Source: CAD feature listing. Evaluate the final solid. Frame: model axes, mm. Round coordinates to 2 decimals unless told otherwise and drop trailing zeros. Write each loop counter-clockwise with the first axis right and the second up, starting at its lowest first coordinate (ties: lowest second). Pieces come first, ordered by that corner, then holes. Notation, with made-up numbers: M -19.5,55.25 L 10.5,55.25 A34 cw 10.5,94.25 Z; hole C 36,47 d2. An arc over 180 degrees is marked long. Answer in a Markdown table with one row per item. Add a question column.
Item 1: Material intervals for probe 1 along X at (y, z) = (1.75, 249); probe 2 along X at (y, z) = (2.4, 26); probe 3 along X at (y, z) = (0.55, -40), sorted ascending.
Item 2: Cut plane D-D on x = 187.5. Return loops of the section in (y, z), and give its area (3 significant figures).
Item 3: Contact query for a flat-ended pin moving along its axis: pin 1 (1.5 mm diameter, centred on x = 364.5, y = 0.5, fed in from -Z). Output: stop coordinate, or through.
Item 4: Cut plane B-B on x = 463. Return loops of the section in (y, z).
Item 5: Mould query, pull axis X, two halves, no side actions, for faces 1 (the face through (19.52, 2.03, 62)), 2 (the face through (271.15, 1.972, 478.537)), 3 (the face through (-271.15, 1.972, -478.537)). Classes: released by +X, released by -X, zero draft, split by the parting line, or undercut.
Item 6: Cut plane A-A on z = 0. Return loops of the section in (x, y).
Item 7: Cut plane C-C on y = 0.95. Give the number of separate pieces and of enclosed holes in the cut face, and give its area (3 significant figures).
from build123d import *

# Parameters (mm, degrees)
BOSS_EXTRUDE1_DEPTH = 4
CUT_EXTRUDE1_REACH  = 842.148
SKETCH3_R           = 4
CUT_EXTRUDE2_REACH  = 842.148
SKETCH4_R           = 3.1
CIRPATTERN1_COUNT   = 6
CUT_EXTRUDE3_REACH  = 842.148
SKETCH5_R           = 65


with BuildPart() as part:
    # Sketch1 → Boss-Extrude1 (new body)
    with BuildSketch(Plane(origin=(0, 0, 0), x_dir=(1, 0, 0), z_dir=(0, 1, 0))):
        Polygon((0, 635.085296109), (-550, 317.542648054), (-550, -317.542648054), (0, -635.085296109), (550, -317.542648054), (550, 317.542648054), align=None)
    extrude(amount=BOSS_EXTRUDE1_DEPTH)

    # Sketch3 → Cut-Extrude1 (cut, up to next)
    with BuildSketch(Plane(origin=(0, 4, 0), x_dir=(1, 0, 0), z_dir=(0, 1, 0)), mode=Mode.PRIVATE) as cut_extrude1_sk1:
        with Locations(Location((53.101090522, 102.006245815, 0), (0, 0, 270))):
            Circle(SKETCH3_R)
    cut_extrude1_tool1 = extrude(cut_extrude1_sk1.sketch, amount=-CUT_EXTRUDE1_REACH, mode=Mode.PRIVATE) & part.part
    # Sketch3 → Cut-Extrude1 (cut, up to next)
    with BuildSketch(Plane(origin=(0, 4, 0), x_dir=(1, 0, 0), z_dir=(0, 1, 0)), mode=Mode.PRIVATE) as cut_extrude1_sk2:
        with Locations(Location((109.677449336, 34.581166943, 0), (0, 0, 270))):
            Circle(SKETCH3_R)
    cut_extrude1_tool2 = extrude(cut_extrude1_sk2.sketch, amount=-CUT_EXTRUDE1_REACH, mode=Mode.PRIVATE) & part.part
    # Sketch3 → Cut-Extrude1 (cut, up to next)
    with BuildSketch(Plane(origin=(0, 4, 0), x_dir=(1, 0, 0), z_dir=(0, 1, 0)), mode=Mode.PRIVATE) as cut_extrude1_sk3:
        with Locations(Location((102.006245815, -53.101090522, 0), (0, 0, 270))):
            Circle(SKETCH3_R)
    cut_extrude1_tool3 = extrude(cut_extrude1_sk3.sketch, amount=-CUT_EXTRUDE1_REACH, mode=Mode.PRIVATE) & part.part
    # Sketch3 → Cut-Extrude1 (cut, up to next)
    with BuildSketch(Plane(origin=(0, 4, 0), x_dir=(1, 0, 0), z_dir=(0, 1, 0)), mode=Mode.PRIVATE) as cut_extrude1_sk4:
        with Locations(Location((34.581166943, -109.677449336, 0), (0, 0, 270))):
            Circle(SKETCH3_R)
    cut_extrude1_tool4 = extrude(cut_extrude1_sk4.sketch, amount=-CUT_EXTRUDE1_REACH, mode=Mode.PRIVATE) & part.part
    # Sketch3 → Cut-Extrude1 (cut, up to next)
    with BuildSketch(Plane(origin=(0, 4, 0), x_dir=(1, 0, 0), z_dir=(0, 1, 0)), mode=Mode.PRIVATE) as cut_extrude1_sk5:
        with Locations(Location((-53.101090522, -102.006245815, 0), (0, 0, 270))):
            Circle(SKETCH3_R)
    cut_extrude1_tool5 = extrude(cut_extrude1_sk5.sketch, amount=-CUT_EXTRUDE1_REACH, mode=Mode.PRIVATE) & part.part
    # Sketch3 → Cut-Extrude1 (cut, up to next)
    with BuildSketch(Plane(origin=(0, 4, 0), x_dir=(1, 0, 0), z_dir=(0, 1, 0)), mode=Mode.PRIVATE) as cut_extrude1_sk6:
        with Locations(Location((-109.677449336, -34.581166943, 0), (0, 0, 270))):
            Circle(SKETCH3_R)
    cut_extrude1_tool6 = extrude(cut_extrude1_sk6.sketch, amount=-CUT_EXTRUDE1_REACH, mode=Mode.PRIVATE) & part.part
    # Sketch3 → Cut-Extrude1 (cut, up to next)
    with BuildSketch(Plane(origin=(0, 4, 0), x_dir=(1, 0, 0), z_dir=(0, 1, 0)), mode=Mode.PRIVATE) as cut_extrude1_sk7:
        with Locations(Location((-102.006245815, 53.101090522, 0), (0, 0, 270))):
            Circle(SKETCH3_R)
    cut_extrude1_tool7 = extrude(cut_extrude1_sk7.sketch, amount=-CUT_EXTRUDE1_REACH, mode=Mode.PRIVATE) & part.part
    # Sketch3 → Cut-Extrude1 (cut, up to next)
    with BuildSketch(Plane(origin=(0, 4, 0), x_dir=(1, 0, 0), z_dir=(0, 1, 0)), mode=Mode.PRIVATE) as cut_extrude1_sk8:
        with Locations(Location((-34.581166943, 109.677449336, 0), (0, 0, 270))):
            Circle(SKETCH3_R)
    cut_extrude1_tool8 = extrude(cut_extrude1_sk8.sketch, amount=-CUT_EXTRUDE1_REACH, mode=Mode.PRIVATE) & part.part
    add(cut_extrude1_tool1.solids().sort_by_distance((53.101091, 4, -102.006246))[0], mode=Mode.SUBTRACT)
    add(cut_extrude1_tool2.solids().sort_by_distance((109.677449, 4, -34.581167))[0], mode=Mode.SUBTRACT)
    add(cut_extrude1_tool3.solids().sort_by_distance((102.006246, 4, 53.101091))[0], mode=Mode.SUBTRACT)
    add(cut_extrude1_tool4.solids().sort_by_distance((34.581167, 4, 109.677449))[0], mode=Mode.SUBTRACT)
    add(cut_extrude1_tool5.solids().sort_by_distance((-53.101091, 4, 102.006246))[0], mode=Mode.SUBTRACT)
    add(cut_extrude1_tool6.solids().sort_by_distance((-109.677449, 4, 34.581167))[0], mode=Mode.SUBTRACT)
    add(cut_extrude1_tool7.solids().sort_by_distance((-102.006246, 4, -53.101091))[0], mode=Mode.SUBTRACT)
    add(cut_extrude1_tool8.solids().sort_by_distance((-34.581167, 4, -109.677449))[0], mode=Mode.SUBTRACT)

    # Sketch4 → Cut-Extrude2 (cut, up to next)
    with BuildSketch(Plane(origin=(0, 4, 0), x_dir=(1, 0, 0), z_dir=(0, 1, 0)), mode=Mode.PRIVATE) as cut_extrude2_sk1:
        with Locations(Location((25.980762114, 608.538290725, 0), (0, 0, 270))):
            Circle(SKETCH4_R)
    cut_extrude2_tool1 = extrude(cut_extrude2_sk1.sketch, amount=-CUT_EXTRUDE2_REACH, mode=Mode.PRIVATE) & part.part
    # Sketch4 → Cut-Extrude2 (cut, up to next)
    with BuildSketch(Plane(origin=(0, 4, 0), x_dir=(1, 0, 0), z_dir=(0, 1, 0)), mode=Mode.PRIVATE) as cut_extrude2_sk2:
        with Locations(Location((51.961524227, 593.538290725, 0), (0, 0, 270))):
            Circle(SKETCH4_R)
    cut_extrude2_tool2 = extrude(cut_extrude2_sk2.sketch, amount=-CUT_EXTRUDE2_REACH, mode=Mode.PRIVATE) & part.part
    # Sketch4 → Cut-Extrude2 (cut, up to next)
    with BuildSketch(Plane(origin=(0, 4, 0), x_dir=(1, 0, 0), z_dir=(0, 1, 0)), mode=Mode.PRIVATE) as cut_extrude2_sk3:
        with Locations(Location((-51.961524227, 593.538290725, 0), (0, 0, 270))):
            Circle(SKETCH4_R)
    cut_extrude2_tool3 = extrude(cut_extrude2_sk3.sketch, amount=-CUT_EXTRUDE2_REACH, mode=Mode.PRIVATE) & part.part
    # Sketch4 → Cut-Extrude2 (cut, up to next)
    with BuildSketch(Plane(origin=(0, 4, 0), x_dir=(1, 0, 0), z_dir=(0, 1, 0)), mode=Mode.PRIVATE) as cut_extrude2_sk4:
        with Locations(Location((-25.980762114, 608.538290725, 0), (0, 0, 270))):
            Circle(SKETCH4_R)
    cut_extrude2_tool4 = extrude(cut_extrude2_sk4.sketch, amount=-CUT_EXTRUDE2_REACH, mode=Mode.PRIVATE) & part.part
    cut_extrude2_1 = cut_extrude2_tool1.solids().sort_by_distance((25.980762, 4, -608.538291))[0]
    add(cut_extrude2_1, mode=Mode.SUBTRACT)
    cut_extrude2_2 = cut_extrude2_tool2.solids().sort_by_distance((51.961524, 4, -593.538291))[0]
    add(cut_extrude2_2, mode=Mode.SUBTRACT)
    cut_extrude2_3 = cut_extrude2_tool3.solids().sort_by_distance((-51.961524, 4, -593.538291))[0]
    add(cut_extrude2_3, mode=Mode.SUBTRACT)
    cut_extrude2_4 = cut_extrude2_tool4.solids().sort_by_distance((-25.980762, 4, -608.538291))[0]
    add(cut_extrude2_4, mode=Mode.SUBTRACT)
    cut_extrude2 = cut_extrude2_1 + cut_extrude2_2 + cut_extrude2_3 + cut_extrude2_4  # Cut-Extrude2 as one shape, for the pattern or mirror that repeats it

    # CirPattern1: Cut-Extrude2 ×6 about axis
    cirpattern1_axis = Axis((0, 0, 0), (0, 1, 0))
    for i in range(1, CIRPATTERN1_COUNT):
        add(cut_extrude2.rotate(cirpattern1_axis, i * 360 / CIRPATTERN1_COUNT), mode=Mode.SUBTRACT)

    # Sketch5 → Cut-Extrude3 (cut, up to next)
    with BuildSketch(Plane(origin=(0, 4, 0), x_dir=(1, 0, 0), z_dir=(0, 1, 0)), mode=Mode.PRIVATE) as cut_extrude3_sk1:
        with Locations(Location((0, 0, 0), (0, 0, 270))):
            Circle(SKETCH5_R)
    cut_extrude3_tool1 = extrude(cut_extrude3_sk1.sketch, amount=-CUT_EXTRUDE3_REACH, mode=Mode.PRIVATE) & part.part
    add(cut_extrude3_tool1.solids().sort_by_distance((0, 4, 0))[0], mode=Mode.SUBTRACT)


solid = part.part
Results below:
| question | item | result |
|---|---|---|
| 1 | probe 1 | -550 to -541.39, -538.61 to 538.61, 541.39 to 550 |
| 1 | probe 2 | -550 to -59.57, 59.57 to 550 |
| 1 | probe 3 | -550 to -51.23, 51.23 to 550 |
| 2 | outline | M 0,-526.83 L 4,-526.83 L 4,526.83 L 0,526.83 Z |
| 2 | area | 4,210 mm2 |
| 3 | pin 1 | z = -425.07 |
| 4 | outline | M 0,-367.77 L 4,-367.77 L 4,367.77 L 0,367.77 Z |
| 5 | face 1 | undercut |
| 5 | face 2 | released by +X |
| 5 | face 3 | released by -X |
| 6 | outline | M -550,0 L -65,0 L -65,4 L -550,4 Z; M 65,0 L 550,0 L 550,4 L 65,4 Z |
| 7 | separate pieces | 1 |
| 7 | enclosed holes | 33 |
| 7 | area | 1,030,000 mm2 |
